```python
from build123d import *

# Parameters (mm, degrees)
BOSS_EXTRUDE2_DEPTH = 22.225
SKETCH4_W           = 25.4
SKETCH4_H           = 66.675
BOSS_EXTRUDE5_DEPTH = 44.45
CUT_EXTRUDE1_DEPTH  = 189.612103602
SKETCH6_W           = 152.4
SKETCH6_H           = 22.225
BOSS_EXTRUDE6_DEPTH = 66.675
CUT_EXTRUDE2_DEPTH  = 189.612103602
CUT_EXTRUDE3_DEPTH  = 189.612103602
SKETCH9_R           = 12.7
CUT_EXTRUDE4_DEPTH  = 189.612103602
CUT_EXTRUDE5_DEPTH  = 189.612103602


with BuildPart() as part:
    # Sketch1 → Boss-Extrude2 (new body)
    with BuildSketch(Plane(origin=(0, 0, 0), x_dir=(1, 0, 0), z_dir=(0, 1, 0))):
        Polygon((0, 0), (0, 88.9), (25.4, 88.9), (127, 88.9), (152.4, 88.9), (152.4, 0), align=None)
    extrude(amount=BOSS_EXTRUDE2_DEPTH)

    # Sketch4 → Boss-Extrude5 (add)
    with BuildSketch(Plane(origin=(0, 22.225, 0), x_dir=(1, 0, 0), z_dir=(0, 1, 0))):
        with Locations((12.7, 33.3375)):
            Rectangle(SKETCH4_W, SKETCH4_H)
        with Locations((139.7, 33.3375)):
            Rectangle(SKETCH4_W, SKETCH4_H)
    extrude(amount=BOSS_EXTRUDE5_DEPTH)

    # Sketch5 → Cut-Extrude1 (cut, through all)
    with BuildSketch(Plane(origin=(152.4, 0, 0), x_dir=(0, 0, -1), z_dir=(1, 0, 0))):
        Polygon((66.675, 66.675), (0, 22.225), (0, 66.675), align=None)
    extrude(amount=-CUT_EXTRUDE1_DEPTH, mode=Mode.SUBTRACT)

    # Sketch6 → Boss-Extrude6 (add)
    with BuildSketch(Plane(origin=(0, 22.225, 0), x_dir=(1, 0, 0), z_dir=(0, 1, 0))):
        with Locations((76.2, 77.7875)):
            Rectangle(SKETCH6_W, SKETCH6_H)
    extrude(amount=BOSS_EXTRUDE6_DEPTH)

    # Sketch7 → Cut-Extrude2 (cut, through all)
    with BuildSketch(Plane.XY.offset(-66.675)):
        Polygon((152.4, 66.675), (152.4, 88.9), (130.175, 88.9), align=None)
    extrude(amount=-CUT_EXTRUDE2_DEPTH, mode=Mode.SUBTRACT)

    # Sketch8 → Cut-Extrude3 (cut, through all)
    with BuildSketch(Plane.XY.offset(-66.675)):
        Polygon((0, 88.9), (22.225, 88.9), (0, 66.675), align=None)
    extrude(amount=-CUT_EXTRUDE3_DEPTH, mode=Mode.SUBTRACT)

    # Sketch9 → Cut-Extrude4 (cut, through all)
    with BuildSketch(Plane(origin=(0, 22.225, 0), x_dir=(1, 0, 0), z_dir=(0, 1, 0))):
        with Locations(Location((50.8, 44.45, 0), (0, 0, 270))):
            Circle(SKETCH9_R)
        with Locations(Location((101.6, 44.45, 0), (0, 0, 270))):
            Circle(SKETCH9_R)
    extrude(amount=-CUT_EXTRUDE4_DEPTH, mode=Mode.SUBTRACT)

    # Sketch12 → Cut-Extrude5 (cut, through all)
    with BuildSketch(Plane.XY.offset(-66.675)):
        with BuildLine():
            Line((63.5, 68.2625), (88.9, 68.2625))
            ThreePointArc((88.9, 68.2625), (101.6, 55.5625), (88.9, 42.8625))
            Line((88.9, 42.8625), (63.5, 42.8625))
            ThreePointArc((63.5, 42.8625), (50.8, 55.5625), (63.5, 68.2625))
        make_face()
    extrude(amount=-CUT_EXTRUDE5_DEPTH, mode=Mode.SUBTRACT)


solid = part.part
```
Geometry check sheet. Reference: the model listing, model coordinates, mm. A direction names the side the tool comes from. Give positions to 0.01 mm unless a question says otherwise; leave off trailing zeros. Loops run counter-clockwise (first coordinate to the right, second up) from the corner with the lowest first, then second, coordinate; pieces in that order, holes last. Notation, with made-up numbers: (21.5, 52.25) - (34.5, 52.25) arc R28 cw to (34.5, 71.25) - close; hole circle Ø9 at (87.5, 44). An arc over 180 degrees is marked (long way). Use CSV: the item, a comma, the result in double quotes. Start each with the question number.
Q1. Section check B-B, the plane x = 96. Record the cut outline in (y, z) (3 decimals).
Q2. Scan lines: probe 1 along X at (y, z) = (12.5, -44.45); probe 2 along Z at (x, y) = (50, 17); probe 3 along X at (y, z) = (38.5, -64). Record each from-to range of solid material in increasing order. Write a range as from..to.
Q3. Access from +Z, -Z, +X, -X, +Y, -Y to the whole of each face (thin tool, end or side, straight path). Record for faces 1 (the face through (50.803, 55.283, -77.632)), 2 (the face through (77, 22.225, -34)), 3 (the face through (77, 0, -45)).
Q4. Section check C-C, the plane z = -44.45. Record the cut outline in (x, y) (3 decimals).
Q5. Section check A-A, the plane z = -78.5. Record the cut outline in (x, y) (1 decimal), and give its area (3 significant figures).
Q6. Go/stop test with flat-tipped pins: pin 1 Ø24.5 at (x, z) = (76.5, -73) entering from -Y; pin 2 Ø4 at (x, y) = (22.5, 59.5) entering from +Z; pin 3 Ø10 at (x, z) = (29, -33) entering from +Y; pin 4 Ø20.5 at (x, z) = (50.8, -44.45) entering from +Y. Record where each tip stops, or that it passes through.
Q7. Section check D-D, the plane y = 62. Record the cut outline in (x, z) (1 decimal), and give its area (3 significant figures).
Q8. Release check for a two-part mould opening along Y. For faces 4 (the face through (76, 42.862, -78)), 5 (the face through (75, 88.9, -78)), 6 (the face through (101.597, 55.842, -77.632)), 7 (the face through (114.192, 11.268, -46.103)) record: +Y half, -Y half, draft (parallel to the pull), parting line (faces both ways), or undercut.
Findings below:
1,outline,"(0, -88.9) - (45.033, -88.9) - (45.033, -66.675) - (22.225, -66.675) - (22.225, -55.849) - (0, -55.849) - close; (0, -33.051) - (22.225, -33.051) - (22.225, 0) - (0, 0) - close; (66.092, -88.9) - (88.9, -88.9) - (88.9, -66.675) - (66.092, -66.675) - close"
2,probe 1,"x = 0..38.1, 63.5..88.9, 114.3..152.4"
2,probe 2,"z = -88.9..-57.12, -31.78..0"
2,probe 3,"x = 0..25.4, 127..152.4"
3,face 1,"+Z, -Z"
3,face 2,"+Z, +Y"
3,face 3,"+Z, -Z, +X, -X, -Y"
4,outline,"(0, 0) - (38.1, 0) - (38.1, 22.225) - (25.4, 22.225) - (25.4, 51.858) - (0, 51.858) - close; (63.5, 0) - (88.9, 0) - (88.9, 22.225) - (63.5, 22.225) - close; (114.3, 0) - (152.4, 0) - (152.4, 51.858) - (127, 51.858) - (127, 22.225) - (114.3, 22.225) - close"
5,outline,"(0, 0) - (152.4, 0) - (152.4, 66.7) - (130.2, 88.9) - (22.2, 88.9) - (0, 66.7) - close; hole (63.5, 42.9) - (88.9, 42.9) arc R12.7 ccw to (88.9, 68.3) - (63.5, 68.3) arc R12.7 ccw to start"
5,area,"11,900 mm^2"
6,pin 1,"stops at y = 0"
6,pin 2,"stops at z = -52.91"
6,pin 3,"stops at y = 46.54"
6,pin 4,"passes through"
7,outline,"(0, -88.9) - (52.6, -88.9) - (52.6, -66.7) - (25.4, -66.7) - (25.4, -59.7) - (0, -59.7) - close; (99.8, -88.9) - (152.4, -88.9) - (152.4, -59.7) - (127, -59.7) - (127, -66.7) - (99.8, -66.7) - close"
7,area,"2,690 mm^2"
8,face 4,"undercut"
8,face 5,"+Y half"
8,face 6,"undercut"
8,face 7,"draft"
